from build123d import *

# Parameters (mm, degrees)
SKETCH_1_W               = 47
SKETCH_1_H               = 39
EXTRUDE_1_DEPTH          = 28
SKETCH_4_W               = 42
SKETCH_4_H               = 34
CUT_EXTRUDE_1_DEPTH      = 25
FILLET_1_R               = 4
HOLE_WIZARD_M2_5_1_D     = 2.05
HOLE_WIZARD_M2_5_1_DEPTH = 6.35
HOLE_WIZARD_M2_5_1_TIP   = 0.615882135
HOLE_WIZARD_M3_1_D       = 2.5
CUT_EXTRUDE_2_REACH      = 41.465
SKETCH_10_R              = 6
SKETCH_11_W              = 7
SKETCH_11_H              = 11
EXTRUDE_2_DEPTH          = 28
HOLE_WIZARD_M4_1_D       = 4.3
CHAMFER_1_SIZE           = 8


with BuildPart() as part:
    # 草图1 → 凸台-拉伸1 (new body)
    with BuildSketch(Plane.XY):
        Rectangle(SKETCH_1_W, SKETCH_1_H)
    extrude(amount=EXTRUDE_1_DEPTH)

    # 草图4 → 切除-拉伸1 (cut)
    with BuildSketch(Plane.XY.offset(28)):
        Rectangle(SKETCH_4_W, SKETCH_4_H)
    extrude(amount=-CUT_EXTRUDE_1_DEPTH, mode=Mode.SUBTRACT)

    # 圆角1
    fillet_1_edges = [part.edges().sort_by_distance(p)[0] for p in [
        (-21, 17, 15.5),
        (-21, -17, 15.5),
        (21, -17, 15.5),
        (21, 17, 15.5),
    ]]
    fillet(fillet_1_edges, radius=FILLET_1_R)

    # M2.5 螺纹孔1
    with Locations(Plane.XY.offset(28)):
        with Locations((21, 17), (-21, -17), (-21, 17), (21, -17)):
            Hole(HOLE_WIZARD_M2_5_1_D / 2, depth=HOLE_WIZARD_M2_5_1_DEPTH)
            with Locations((0, 0, -(HOLE_WIZARD_M2_5_1_DEPTH + HOLE_WIZARD_M2_5_1_TIP / 2))):  # 118° drill point
                Cone(0, HOLE_WIZARD_M2_5_1_D / 2, HOLE_WIZARD_M2_5_1_TIP, mode=Mode.SUBTRACT)

    # M3 螺纹孔1 (through all)
    with Locations(Plane(origin=(0, 0, 0), x_dir=(-1, 0, 0), z_dir=(0, 0, -1))):
        with Locations((-12, -6.5), (12, -6.5), (0, 10.5)):
            Hole(HOLE_WIZARD_M3_1_D / 2)

    # 草图10 → 切除-拉伸2 (cut, up to next)
    with BuildSketch(Plane.XY.offset(3), mode=Mode.PRIVATE) as cut_extrude_2_sk1:
        Circle(SKETCH_10_R)
    cut_extrude_2_tool1 = extrude(cut_extrude_2_sk1.sketch, amount=-CUT_EXTRUDE_2_REACH, mode=Mode.PRIVATE) & part.part
    add(cut_extrude_2_tool1.solids().sort_by_distance((0, 0, 3))[0], mode=Mode.SUBTRACT)

    # 草图11 → 凸台-拉伸2 (add)
    with BuildSketch(Plane(origin=(0, 0, 0), x_dir=(-1, 0, 0), z_dir=(0, 0, -1))):
        with Locations((0, 25)):
            Rectangle(SKETCH_11_W, SKETCH_11_H)
    extrude(amount=-EXTRUDE_2_DEPTH)

    # M4 间隙孔1 (through all)
    with Locations(Plane(origin=(3.5, 0, 0), x_dir=(0, 0, -1), z_dir=(1, 0, 0))):
        with Locations((-15, 26.5)):
            Hole(HOLE_WIZARD_M4_1_D / 2)

    # 倒角1
    chamfer_1_edges = [part.edges().sort_by_distance(p)[0] for p in [
        (0, 30.5, 28),
        (0, 30.5, 0),
    ]]
    chamfer(chamfer_1_edges, length=CHAMFER_1_SIZE)


solid = part.part
Can you work these out from the model? Positions are in its coordinate system, mm. A direction names the side the tool comes from. Round coordinates to 2 decimals unless told otherwise and drop trailing zeros. Order: outer loops, then holes, each group sorted by start corner. A loop starts at its lowest first (then second) coordinate and runs counter-clockwise, first axis right, second up. Notation, with made-up numbers: M -22,87.5 L 14,87.5 A13 ccw 14,104.5 Z; hole C -30.5,82.5 d11. An arc over 180 degrees is marked long. Use a Markdown table: item, result.
1) If I drill on line 1 along Y through (x, z) = (12, 18.5); line 2 along Y through (x, z) = (12, 1.7); line 3 along X through (y, z) = (-1.5, 7.5), over which ranges is the centre line in solid material (lowest first)?
Geometry says:
| item | result |
|---|---|
| line 1 | y = -19.5 to -17, 17 to 19.5 |
| line 2 | y = -19.5 to -7.75, -5.25 to 19.5 |
| line 3 | x = -23.5 to -21, 21 to 23.5 |
2) Imagine slicing it at A-A (x = 0). List the corners of the cut face in (y, z) for me, then the cut area to 3 significant figures.
Geometry says:
| item | result |
|---|---|
| outline | M -19.5,0 L -6,0 L -6,3 L -17,3 L -17,28 L -19.5,28 Z; M 6,0 L 9.25,0 L 9.25,3 L 6,3 Z; M 11.75,0 L 22.5,0 L 30.5,8 L 30.5,20 L 22.5,28 L 17,28 L 17,3 L 11.75,3 Z; hole C 26.5,15 d4.3 |
| area | 428 mm² |
3) Imagine slicing it at D-D (z = 10). List the corners of the cut face in (x, y) for me, then the cut area to 3 significant figures.
Geometry says:
| item | result |
|---|---|
| outline | M -23.5,-19.5 L 23.5,-19.5 L 23.5,19.5 L 3.5,19.5 L 3.5,30.5 L -3.5,30.5 L -3.5,19.5 L -23.5,19.5 Z; hole M -21,-13 A4 ccw -17,-17 L 17,-17 A4 ccw 21,-13 L 21,13 A4 ccw 17,17 L -17,17 A4 ccw -21,13 Z |
| area | 496 mm² |
4) I'm going to push flat-ended pins straight in: P1, Ø2, axis at x = -16, z = 12.5, coming from the +Y side; P2, Ø2, axis at y = 22, z = 21.5, coming from the +X side; P3, Ø9, axis at y = 27, z = 17, coming from the -X side. Where does each tip first touch, or does it pass through?
Geometry says:
| item | result |
|---|---|
| P1 | stops at y = 19.5 |
| P2 | stops at x = 3.5 |
| P3 | stops at x = -3.5 |
5) Imagine slicing it at C-C (z = 24). List the corners of the cut face in (x, y) for me (3 decimals).
Geometry says:
| item | result |
|---|---|
| outline | M -23.5,-19.5 L 23.5,-19.5 L 23.5,19.5 L 3.5,19.5 L 3.5,26.5 L -3.5,26.5 L -3.5,19.5 L -23.5,19.5 Z; hole C -21,-17 d2.05; hole C -21,17 d2.05; hole M -21,-13 A4 ccw -17,-17 L 17,-17 A4 ccw 21,-13 L 21,13 A4 ccw 17,17 L -17,17 A4 ccw -21,13 Z; hole C 21,-17 d2.05; hole C 21,17 d2.05 |
6) If we mould it in two halves opening along Y, with no side actions, what happens to faces 3 (the face through (0, -19.5, 14)), 4 (the face through (-0.16, 11.74, 1.52)), 5 (the face through (-14, 19.5, 14))? For each: +Y half, -Y half, draft (parallel to the pull), parting line (faces both ways), or undercut.
Geometry says:
| item | result |
|---|---|
| face 3 | -Y half |
| face 4 | undercut |
| face 5 | +Y half |
7) Imagine slicing it at B-B (y = 10.5). List the corners of the cut face in (x, z) for me, then the cut area to 4 significant figures.
Geometry says:
| item | result |
|---|---|
| outline | M -23.5,0 L -1.25,0 L -1.25,3 L -21,3 L -21,28 L -23.5,28 Z; M 1.25,0 L 23.5,0 L 23.5,28 L 21,28 L 21,3 L 1.25,3 Z |
| area | 258.5 mm² |
8) On a 3-axis mill with a long thin cutter (end or side, diameter ignored), from which of +Z, -Z, +X, -X, +Y, -Y can I reach the whole of each face in a straight line? I mean faces 1 (the face through (-6, -3, 0)), 2 (the face through (0, -17, 16)). Say none if no direction works.
Geometry says:
| item | result |
|---|---|
| face 1 | -Z, +X, -X, +Y, -Y |
| face 2 | +Z |
